For this review, take the finished solid that the model builds, in its own axes (mm). A direction names the side the tool comes from. Give positions to 0.01 mm unless a question says otherwise; leave off trailing zeros. Write each loop counter-clockwise with the first axis right and the second up, starting at its lowest first coordinate (ties: lowest second). Pieces come first, ordered by that corner, then holes. Notation, with made-up numbers: (50.25, 72) -> (78.25, 72) arc R11 cw to (78.25, 80) -> close; hole circle Ø9 at (22.25, 48.25). An arc over 180 degrees is marked (long way). Answer as CSV lines item,"result".
```python
from build123d import *

# Parameters (mm, degrees)
F0_W      = 88.9
F0_H      = 38.1
F1_DEPTH  = 50.8
F2_W      = 12.7
F2_H      = 25.4
F3_DEPTH  = 50.801
F4_W      = 25.4
F4_H      = 25.4
F5_DEPTH  = 50.801
F6_W      = 50.8
F6_H      = 12.7
F7_DEPTH  = 6.35
F8_W      = 12.7
F8_H      = 12.7
F9_DEPTH  = 6.35
F10_W     = 12.7
F10_H     = 12.7
F11_DEPTH = 6.35
F12_R     = 6.35
F13_DEPTH = 50.801


with BuildPart() as f1:
    # F0 (on Front) → F1 (new body)
    with BuildSketch(Plane.XZ):
        Rectangle(F0_W, F0_H)
    extrude(amount=F1_DEPTH)

    # F2 (on face) → F3 (cut, through all)
    with BuildSketch(Plane.XZ.offset(50.8)):
        with Locations((-38.1, 6.35)):
            Rectangle(F2_W, F2_H)
    extrude(amount=-F3_DEPTH, mode=Mode.SUBTRACT)

    # F4 (on face) → F5 (cut, through all)
    with BuildSketch(Plane.XZ.offset(50.8)):
        with Locations((31.75, 6.35)):
            Rectangle(F4_W, F4_H)
    extrude(amount=-F5_DEPTH, mode=Mode.SUBTRACT)

    # F6 (on face) → F7 (join)
    with BuildSketch(Plane.XY.offset(19.05)):
        with Locations((-6.35, -6.35)):
            Rectangle(F6_W, F6_H)
        with Locations((-6.35, -44.45)):
            Rectangle(F6_W, F6_H)
    extrude(amount=F7_DEPTH)

    # F8 (on face) → F9 (join)
    with BuildSketch(Plane.XY.offset(25.4)):
        with Locations((-25.4, -6.35)):
            Rectangle(F8_W, F8_H)
        with Locations((12.7, -6.35)):
            Rectangle(F8_W, F8_H)
    extrude(amount=F9_DEPTH)

    # F10 (on face) → F11 (join)
    with BuildSketch(Plane.XY.offset(25.4)):
        with Locations((-25.4, -44.45)):
            Rectangle(F10_W, F10_H)
        with Locations((12.7, -44.45)):
            Rectangle(F10_W, F10_H)
    extrude(amount=F11_DEPTH)

    # F12 (on face) → F13 (cut, through all)
    with BuildSketch(Plane.XZ.offset(50.8)):
        with Locations((-6.35, -6.35)):
            Circle(F12_R)
    extrude(amount=-F13_DEPTH, mode=Mode.SUBTRACT)


solid = f1.part
```
Q1. Add section C-C (z = 23). Write out the cut boundary in (x, y).
Answer block:
outline,"(-31.75, -50.8) -> (19.05, -50.8) -> (19.05, -38.1) -> (-31.75, -38.1) -> close; (-31.75, -12.7) -> (19.05, -12.7) -> (19.05, 0) -> (-31.75, 0) -> close"
Q2. Draft analysis for pull direction Y (two halves, no side actions). For faces 6 (the flat face through (-11, 0, 0)), 7 (the flat face through (-7, -12.7, 24)), 8 (the flat face through (-44.45, -25, -13)), state which applies: released by +Y, released by -Y, zero draft, split by the parting line, or undercut.
Answer block:
face 6,"released by +Y"
face 7,"undercut"
face 8,"zero draft"
Q3. To check wall thickness, follow probe 1 along Z at (x, y) = (-6.35, -34); probe 2 along Y at (x, z) = (-1, 25); probe 3 along Z at (x, y) = (-6.35, -40). State the ranges of each line that lie inside material, in increasing order. Write a range as [from, to].
Answer block:
probe 1,"z = [-19.05, -12.7], [0, 19.05]"
probe 2,"y = [-50.8, -38.1], [-12.7, 0]"
probe 3,"z = [-19.05, -12.7], [0, 25.4]"
Q4. Add section D-D (x = 18). Write out the cut boundary in (y, z), plus the area to 3 significant figures.
Answer block:
outline,"(-50.8, -19.05) -> (0, -19.05) -> (0, 31.75) -> (-12.7, 31.75) -> (-12.7, 19.05) -> (-38.1, 19.05) -> (-38.1, 31.75) -> (-50.8, 31.75) -> close"
area,"2,260 mm2"
Q5. Add section A-A (y = -40). Write out the cut boundary in (x, z), plus the area to 3 significant figures.
Answer block:
outline,"(-44.45, -19.05) -> (44.45, -19.05) -> (44.45, -6.35) -> (19.05, -6.35) -> (19.05, 31.75) -> (6.35, 31.75) -> (6.35, 25.4) -> (-19.05, 25.4) -> (-19.05, 31.75) -> (-31.75, 31.75) -> (-31.75, -6.35) -> (-44.45, -6.35) -> close; hole circle Ø12.7 at (-6.35, -6.35)"
area,"2,780 mm2"
Q6. For faces 1 (the flat face through (-31.75, -26, 8)), 2 (the flat face through (-7, -25, 19.05)), 3 (the flat face through (-1, -25, -19.05)), 4 (the flat face through (-19.05, -6, 29)), 5 (the flat face through (19.05, -26, 8)), list the 3-axis set-ups (+Z, -Z, +X, -X, +Y, -Y) from which the entire face can be reached by the end or side of a thin tool; tool diameter is ignored.
Answer block:
face 1,"+Z, -X, +Y, -Y"
face 2,"+Z, +X, -X"
face 3,"-Z, +X, -X, +Y, -Y"
face 4,"+Z, +Y, -Y"
face 5,"+Z, +X, +Y, -Y"
Q7. Clearance check with flat-ended pins moving along their axes: pin 1 (10 mm diameter, centred on x = -5.5, y = -7.5, fed in from +Z); pin 2 (5 mm diameter, centred on y = -46, z = 28, fed in from +X); pin 3 (1.5 mm diameter, centred on y = -38, z = 3.5, fed in from +X); pin 4 (2 mm diameter, centred on y = -37, z = 20.5, fed in from +X). State where each tip first meets the part, or that it passes through.
Answer block:
pin 1,"stops at z = 25.4"
pin 2,"stops at x = 19.05"
pin 3,"stops at x = 19.05"
pin 4,"passes through"
Q8. Add section B-B (x = -6.35). Write out the cut boundary in (y, z).
Answer block:
outline,"(-50.8, -19.05) -> (0, -19.05) -> (0, -12.7) -> (-50.8, -12.7) -> close; (-50.8, 0) -> (0, 0) -> (0, 25.4) -> (-12.7, 25.4) -> (-12.7, 19.05) -> (-38.1, 19.05) -> (-38.1, 25.4) -> (-50.8, 25.4) -> close"
